from build123d import *

# Parameters (mm, degrees)
F1_DEPTH = 7
F3_ANGLE = 240
F4_ANGLE = 120
F6_R     = 2.5


with BuildPart() as f1:
    # F0 (on Top) → F1 (new body)
    with BuildSketch(Plane.XY):
        with BuildLine():
            ThreePointArc((-11, 0), (-7.7781745931, 7.7781745931), (0, 11))
            Line((0, 11), (0, 15))
            ThreePointArc((0, 15), (-11, 26), (0, 37))
            Line((0, 37), (0, 40))
            Line((0, 40), (-17, 40))
            Line((-17, 40), (-17, 0))
            Line((-17, 0), (-11, 0))
        make_face()
        with BuildLine():
            ThreePointArc((0, 11), (7.7781745931, 7.7781745931), (11, 0))
            Line((11, 0), (17, 0))
            Line((17, 0), (17, 9.8637529312))
            ThreePointArc((17, 9.8637529312), (10.5771972535, 16.2865556777), (17, 22.7093584241))
            Line((17, 22.7093584241), (17, 40))
            Line((17, 40), (0, 40))
            Line((0, 40), (0, 37))
            ThreePointArc((0, 37), (7.7781745931, 33.7781745931), (11, 26))
            ThreePointArc((11, 26), (7.7781745931, 18.2218254069), (0, 15))
            Line((0, 15), (0, 11))
        make_face()
    extrude(amount=F1_DEPTH)


with BuildPart() as f3_1:
    # F3: copy of F1
    add(f1.part.rotate(Axis((0, 0, 24.7764140368), (0, 0, 1)), F3_ANGLE))


with BuildPart() as f4_1:
    # F4: copy of F1
    add(f1.part.rotate(Axis((0, 0, 24.7764140368), (0, 0, 1)), F4_ANGLE))


with BuildPart() as f1_1:
    add(f1.part)

    # F5: union F3_1, F4_1
    add(f3_1.part)
    add(f4_1.part)

    # F6
    f6_edges = [f1_1.edges().sort_by_distance(p)[0] for p in [
        (-17, 24.907477, 7),
        (-17, 24.907477, 0),
        (-35.653949, -0.954908, 7),
        (-35.653949, -0.954908, 0),
        (-13.070508, -27.176171, 7),
        (-13.070508, -27.176171, 0),
        (-34.641016, -20, 7),
        (-34.641016, -20, 0),
    ]]
    fillet(f6_edges, radius=F6_R)


solid = f1_1.part
Input: part model. Units: mm. Frame: model coordinates. A direction names the side the tool comes from. Round coordinates to 2 decimals unless told otherwise and drop trailing zeros. Write each loop counter-clockwise with the first axis right and the second up, starting at its lowest first coordinate (ties: lowest second). Pieces come first, ordered by that corner, then holes.
1) Draft query along X for faces 1 (the flat face through (0, 40, 3)), 2 (the cylindrical face through (11.37, 19.38, 3.45)), 3 (the cylindrical face through (-13.263, -26.419, 6.287)), 4 (the cylindrical face through (-16.248, 24.696, 0.713)). Return one class per face: pulls with the +X half, pulls with the -X half, needs draft (parallel to the pull), parting line crosses it, or undercut.
2) Cut plane A-A (y = 33.5). Return the cut outline in (x, z).
3) Ray query, L1, parallel to Y at x = 9, z = 1.5; L2, parallel to Y at x = -6.5, z = 5.75; L3, parallel to X at y = 10, z = 5.75. Return the intervals inside material, ascending.
4) Contact query for flat-ended pins moving along their axis: P1, Ø3, axis at x = -19.5, z = 2.5, coming from the -Y side; P2, Ø1.6, axis at y = 26, z = 3, coming from the -X side; P3, Ø3, axis at y = -26.5, z = 1, coming from the +X side. Output: stop coordinate, or through.
5) Cut plane B-B (y = -13). Count the separate pieces of the cut face and the enclosed holes in it, then the cut area to 3 significant figures.
6) Cut plane C-C (z = 1.5). Return the cut outline in (x, y), then the cut area to 3 significant figures.
7) Reachability of faces 5 (the cylindrical face through (-16.248, 24.696, 6.287)), 6 (the flat face through (34.52, -20.21, 3.45)), 7 (the flat face through (-17, 25, 3)), 8 (the flat face through (17, 31, 3)), 9 (the flat face through (-13.25, -27.28, 3.49)) from +Z, -Z, +X, -X, +Y, -Y: full face, straight path, thin tool, end or side. Return the list, or none.
Geometry says:
1. face 1: needs draft
1. face 2: pulls with the +X half
1. face 3: undercut
1. face 4: pulls with the -X half
2. outline: (-17, 2.5) arc R2.5 ccw to (-14.5, 0) - (-8.05, 0) - (-8.05, 7) - (-14.5, 7) arc R2.5 ccw to (-17, 4.5) - close; (8.05, 0) - (17, 0) - (17, 7) - (8.05, 7) - close
3. L1: y = -17.41 to -6.32, 6.32 to 19.68, 32.32 to 40
3. L2: y = -23 to -8.87, 8.87 to 17.13, 34.87 to 40
3. L3: x = -16.68 to -4.58, 4.58 to 16.68
4. P1: stops at y = -31.75
4. P2: stops at x = -17
4. P3: stops at x = 31.75
5. separate pieces: 3
5. enclosed holes: 0
5. area: 230 mm2
6. outline: (-42.86, -5.35) - (-26.06, -34.44) - (-0.21, -19.51) - (0.04, -19.65) arc R6.42 cw to (0.09, -19.58) - (5.52, -16.44) arc R6.42 cw to (11.17, -26.08) - (26.14, -34.72) - (43.14, -5.28) - (17, 9.81) - (17, 9.86) arc R6.42 cw to (16.91, 9.86) - (11.48, 13) arc R6.42 cw to (17, 22.71) - (17, 40) - (-16.79, 40) - (-16.79, 9.94) - (-17.04, 9.79) arc R6.42 cw to (-17, 9.72) - (-17, 3.44) arc R6.42 cw to (-28.06, 3.19) - close; hole circle Ø22 at (-22.52, -13); hole circle Ø22 at (0, 0); hole circle Ø22 at (0, 26); hole circle Ø22 at (22.52, -13)
6. area: 1,850 mm2
7. face 5: +Z, -X, +Y
7. face 6: +Z, -Z, +X, -Y
7. face 7: +Z, -Z, -X, +Y
7. face 8: +Z, -Z, +X, +Y
7. face 9: +Z, -Z, -Y
